Answer from the drawing. Dimensions are ordinates in mm from the lowest x, y and z of the part. Round coordinates to 2 decimals unless told otherwise and drop trailing zeros. Order: outer loops, then holes, each group sorted by start corner. A loop starts at its lowest first (then second) coordinate and runs counter-clockwise, first axis right, second up. Notation, with made-up numbers: (4, 79) -> (22, 79) arc R38 cw to (22, 118) -> close; hole circle Ø1 at (-7, 7.25). An arc over 180 degrees is marked (long way). Use a Markdown table: item, result. Add a question column.
Item 1: Find the intervals of material crossed by L1, parallel to X at y = 0.2, z = 11.5; L2, parallel to Z at x = 3.5, y = 0.35; L3, parallel to Z at x = 8.75, y = 0.8, in increasing order. Write a range as [from, to].
Item 2: A cutting plane is placed at D-D, the plane z = 12.75. Determine the outline of the cut face in (x, y).
Item 3: A cutting plane is placed at B-B, the plane y = 0.2. Determine the outline of the cut face in (x, z).
Item 4: A cutting plane is placed at A-A, the plane x = 1.25. Determine the outline of the cut face in (y, z), plus the area to 3 significant figures.
Item 5: A cutting plane is placed at C-C, the plane x = 8.25. Determine the outline of the cut face in (y, z), plus the area to 3 significant figures.
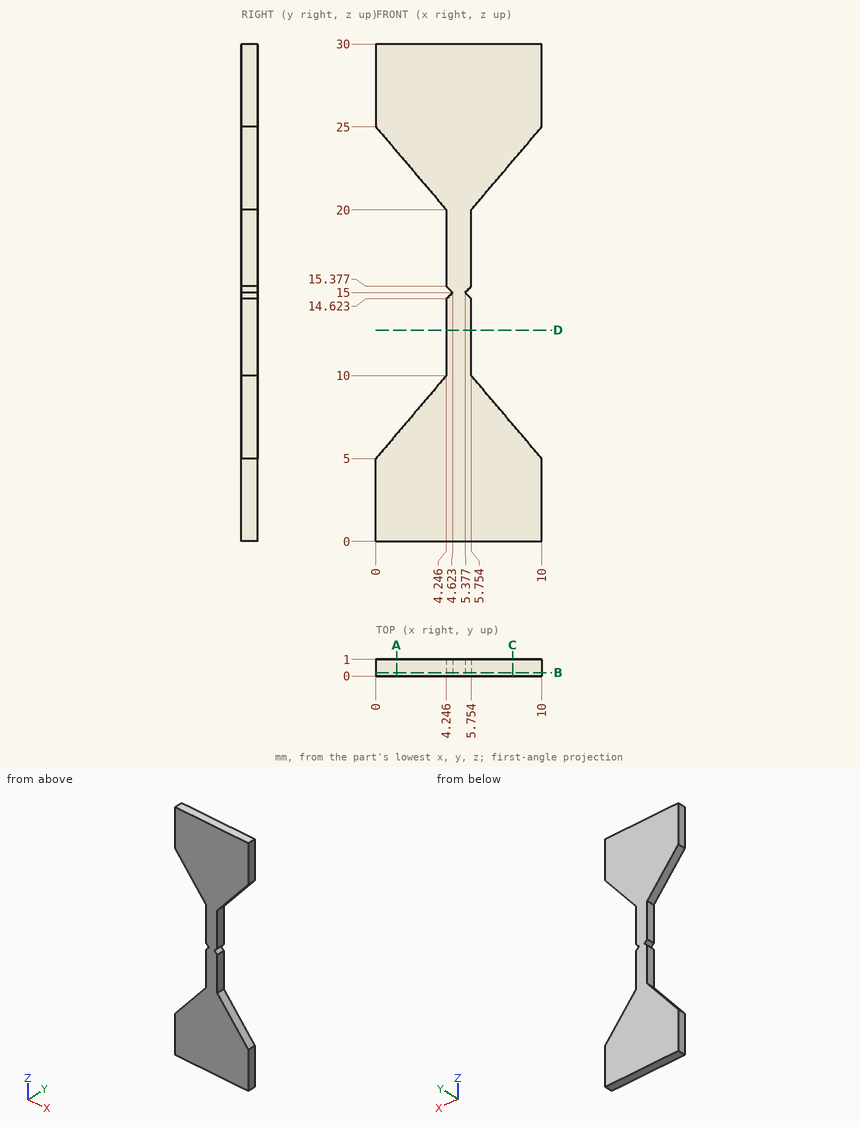
Reported:
| question | item | result |
|---|---|---|
| 1 | L1 | [4.25, 5.75] |
| 1 | L2 | [0, 9.12], [20.88, 30] |
| 1 | L3 | [0, 6.47], [23.53, 30] |
| 2 | outline | (4.25, 0) -> (5.75, 0) -> (5.75, 1) -> (4.25, 1) -> close |
| 3 | outline | (0, 0) -> (10, 0) -> (10, 5) -> (5.75, 10) -> (5.75, 14.62) -> (5.38, 15) -> (5.75, 15.38) -> (5.75, 20) -> (10, 25) -> (10, 30) -> (0, 30) -> (0, 25) -> (4.25, 20) -> (4.25, 15.38) -> (4.62, 15) -> (4.25, 14.62) -> (4.25, 10) -> (0, 5) -> close |
| 4 | outline | (0, 0) -> (1, 0) -> (1, 6.47) -> (0, 6.47) -> close; (0, 23.53) -> (1, 23.53) -> (1, 30) -> (0, 30) -> close |
| 4 | area | 12.9 mm² |
| 5 | outline | (0, 0) -> (1, 0) -> (1, 7.06) -> (0, 7.06) -> close; (0, 22.94) -> (1, 22.94) -> (1, 30) -> (0, 30) -> close |
| 5 | area | 14.1 mm² |
